from build123d import *

# Parameters (mm, degrees)
SKETCH1_W           = 88.9
SKETCH1_H           = 82.55
BOSS_EXTRUDE1_DEPTH = 111.125
SKETCH2_W           = 76.2
SKETCH2_H           = 209.55
CUT_EXTRUDE1_DEPTH  = 76.2
SKETCH3_W           = 38.1
SKETCH3_H           = 6.096
BOSS_EXTRUDE2_DEPTH = 6.35
SKETCH4_W           = 19.05
SKETCH4_H           = 0.762
CUT_EXTRUDE2_DEPTH  = 231.379015158
FILLET1_R           = 6.35
FILLET2_R           = 6.35


with BuildPart() as part:
    # Sketch1 → Boss-Extrude1 (new, symmetric)
    with BuildSketch(Plane.XY):
        Rectangle(SKETCH1_W, SKETCH1_H)
    extrude(amount=BOSS_EXTRUDE1_DEPTH, both=True)

    # Sketch2 → Cut-Extrude1 (cut)
    with BuildSketch(Plane(origin=(0, 41.275, 0), x_dir=(1, 0, 0), z_dir=(0, 1, 0))):
        Rectangle(SKETCH2_W, SKETCH2_H)
    extrude(amount=-CUT_EXTRUDE1_DEPTH, mode=Mode.SUBTRACT)

    # Sketch3 → Boss-Extrude2 (add, symmetric)
    with BuildSketch(Plane.XY.offset(111.125)):
        Rectangle(SKETCH3_W, SKETCH3_H)
    extrude(amount=BOSS_EXTRUDE2_DEPTH, both=True)

    # Sketch4 → Cut-Extrude2 (cut, through all)
    with BuildSketch(Plane.XY.offset(111.125)):
        with Locations((-19.05, -40.894)):
            Rectangle(SKETCH4_W, SKETCH4_H)
        with Locations((19.05, -40.894)):
            Rectangle(SKETCH4_W, SKETCH4_H)
    extrude(amount=-CUT_EXTRUDE2_DEPTH, mode=Mode.SUBTRACT)

    # Fillet1
    fillet1_edges = [part.edges().sort_by_distance(p)[0] for p in [
        (44.45, 0, 111.125),
        (44.45, 0, -111.125),
        (-44.45, 0, -111.125),
        (-44.45, 0, 111.125),
    ]]
    fillet(fillet1_edges, radius=FILLET1_R)

    # Fillet2
    fillet2_edges = [part.edges().sort_by_distance(p)[0] for p in [
        (19.05, 0, 117.475),
        (-19.05, 0, 117.475),
    ]]
    fillet(fillet2_edges, radius=FILLET2_R - 0.0001)  # a hair under: the kernel refuses the full size


solid = part.part
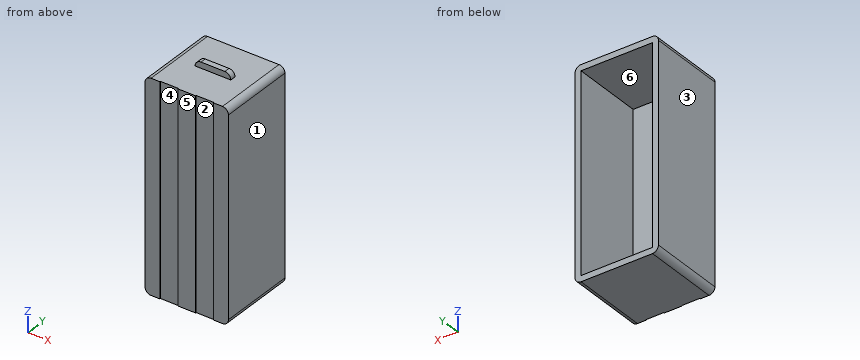
Input: part model. Units: mm. Frame: model coordinates. Face numbers are marked on the shaded views. A direction names the side the tool comes from. Give positions to 0.01 mm unless a question says otherwise; leave off trailing zeros. Write each loop counter-clockwise with the first axis right and the second up, starting at its lowest first coordinate (ties: lowest second). Pieces come first, ordered by that corner, then holes. Notation, with made-up numbers: (61.5, -20.5) -> (106.5, -20.5) arc R19 ccw to (106.5, -10.5) -> close; hole circle Ø3 at (71, -8.5). An arc over 180 degrees is marked (long way). Use one line per item in the form item = value. Start each with the question number.
1) Section query A-A on y = 5.5. Return the cut outline in (x, z) (3 decimals).
2) Section query C-C on x = -32. Return the cut outline in (y, z) (3 decimals), then the cut area to 3 significant figures.
3) Section query D-D on x = -2.5. Return the cut outline in (y, z) (3 decimals), then the cut area to 3 significant figures.
4) Set-up query: the marked faces 5 and 6. Return all of +Z, -Z, +X, -X, +Y, -Y with unobstructed straight access to the full face (end or side cutting, diameter ignored); none if empty.
5) Section query B-B on z = -69.5. Return the cut outline in (x, y) (3 decimals), then the cut area to 3 significant figures.
6) Draft query along X for the marked faces 1, 2, 3 and 4. Return one class per face: pulls with the +X half, pulls with the -X half, needs draft (parallel to the pull), parting line crosses it, or undercut.
7) Pin query (flat end, axial travel): pin 1 (3 mm diameter, centred on x = 4.5, z = 114.5, fed in from +Y); pin 2 (2 mm diameter, centred on x = -7, z = 30, fed in from +Y) (3 decimals); pin 3 (5 mm diameter, centred on x = 18.5, y = -25.5, fed in from +Z) (3 decimals). Return the tip coordinate at first contact, or that it passes through.
8) Ray query, probe 1 along X at (y, z) = (14.5, 58); probe 2 along Z at (x, y) = (5.5, 31) (3 decimals); probe 3 along Y at (x, z) = (38, 23.5) (3 decimals). Return the intervals inside material, ascending. Write a range as from..to.
Outcome:
q1.outline = (-44.45, -104.775) arc R6.35 ccw to (-38.1, -111.125) -> (38.1, -111.125) arc R6.35 ccw to (44.45, -104.775) -> (44.45, 104.775) arc R6.35 ccw to (38.1, 111.125) -> (-38.1, 111.125) arc R6.35 ccw to (-44.45, 104.775) -> close; hole (-38.1, -104.775) -> (38.1, -104.775) -> (38.1, 104.775) -> (-38.1, 104.775) -> close
q2.outline = (-41.275, -111.125) -> (41.275, -111.125) -> (41.275, -104.775) -> (-34.925, -104.775) -> (-34.925, 104.775) -> (41.275, 104.775) -> (41.275, 111.125) -> (-41.275, 111.125) -> close
q2.area = 2,380 mm^2
q3.outline = (-41.275, -111.125) -> (41.275, -111.125) -> (41.275, -104.775) -> (-34.925, -104.775) -> (-34.925, 104.775) -> (41.275, 104.775) -> (41.275, 111.125) -> (3.048, 111.125) -> (3.048, 117.475) -> (-3.048, 117.475) -> (-3.048, 111.125) -> (-41.275, 111.125) -> close
q3.area = 2,420 mm^2
q4.face_5 = +Z, -Z, +X, -X, -Y
q4.face_6 = +Y
q5.outline = (-44.45, -41.275) -> (-28.575, -41.275) -> (-28.575, -40.513) -> (-9.525, -40.513) -> (-9.525, -41.275) -> (9.525, -41.275) -> (9.525, -40.513) -> (28.575, -40.513) -> (28.575, -41.275) -> (44.45, -41.275) -> (44.45, 41.275) -> (38.1, 41.275) -> (38.1, -34.925) -> (-38.1, -34.925) -> (-38.1, 41.275) -> (-44.45, 41.275) -> close
q5.area = 1,500 mm^2
q6.face_1 = pulls with the +X half
q6.face_2 = undercut
q6.face_3 = pulls with the -X half
q6.face_4 = undercut
q7.pin_1 = 3.05
q7.pin_2 = -34.925
q7.pin_3 = 111.125
q8.probe_1 = -44.45..-38.1, 38.1..44.45
q8.probe_2 = -111.125..-104.775, 104.775..111.125
q8.probe_3 = -41.275..-34.925
